The model under review builds one solid part; all positions refer to its coordinate system, in mm. A direction names the side the tool comes from. Coordinates: 2 decimals unless noted, no trailing zeros. Loops run counter-clockwise (first coordinate to the right, second up) from the corner with the lowest first, then second, coordinate; pieces in that order, holes last. Notation, with made-up numbers: (-11, 19.5) - (25, 19.5) arc R22 ccw to (25, 29.5) - close; hole circle Ø6 at (20.5, -18). An arc over 180 degrees is marked (long way). Use a Markdown table: item, result. Add a question column.
1) To check wall thickness, follow L1, parallel to Y at x = 0, z = 41.5; L2, parallel to Z at x = -29, y = 24; L3, parallel to X at y = -3.5, z = 76. State the ranges of each line that lie inside material, in increasing order. Write a range as [from, to].
2) Add section C-C, the plane y = -35. Give the boundary of the cut face in (x, z), and give its area (3 significant figures).
3) For faces 1 (the cylindrical face through (-32.798, 30.075, 62.84)), 2 (the flat face through (9, -19, 0)), list the 3-axis set-ups (+Z, -Z, +X, -X, +Y, -Y) from which the entire face can be reached by the end or side of a thin tool; tool diameter is ignored.
4) Add section D-D, the plane z = 34.5. Give the boundary of the cut face in (x, y), and give its area (3 significant figures).
5) Clearance check with flat-ended pins moving along their axes: pin 1 (1.5 mm diameter, centred on x = -23.5, y = 25, fed in from +Z); pin 2 (6 mm diameter, centred on x = 14, z = 45.5, fed in from -Y); pin 3 (12 mm diameter, centred on x = 35.5, z = 55, fed in from +Y). State where each tip first meets the part, or that it passes through.
6) Add section A-A, the plane x = 0. Give the boundary of the cut face in (y, z), and give its area (3 significant figures).
```python
from build123d import *

# Parameters (mm, degrees)
F0_R        = 45
F0_R_2      = 20
F1_DEPTH    = 2
F1_FACE_R   = 45
F1_FACE_R_2 = 20
F2_DEPTH    = 120
F3_R        = 44.5
F4_DEPTH    = 120


with BuildPart() as f1:
    # F0 (on Top) → F1 (new body)
    with BuildSketch(Plane.XY):
        Circle(F0_R)
        Circle(F0_R_2, mode=Mode.SUBTRACT)
    extrude(amount=F1_DEPTH)

    # F1_face (on face) → F2 (join)
    with BuildSketch(Plane.XY.offset(2)):
        Circle(F1_FACE_R)
        Circle(F1_FACE_R_2, mode=Mode.SUBTRACT)
    extrude(amount=F2_DEPTH)

    # F3 (on face) → F4 (cut)
    with BuildSketch(Plane.XY.offset(122)):
        Circle(F3_R)
    extrude(amount=-F4_DEPTH, mode=Mode.SUBTRACT)


solid = f1.part
```
From the geometry:
| question | item | result |
|---|---|---|
| 1 | L1 | y = [-45, -44.5], [44.5, 45] |
| 1 | L2 | z = [0, 2] |
| 1 | L3 | x = [-44.86, -44.36], [44.36, 44.86] |
| 2 | outline | (-28.28, 0) - (28.28, 0) - (28.28, 122) - (27.48, 122) - (27.48, 2) - (-27.48, 2) - (-27.48, 122) - (-28.28, 122) - close |
| 2 | area | 306 mm^2 |
| 3 | face 1 | +Z |
| 3 | face 2 | -Z, +X, -X, +Y, -Y |
| 4 | outline | circle Ø90 at (0, 0); hole circle Ø89 at (0, 0) |
| 4 | area | 141 mm^2 |
| 5 | pin 1 | stops at z = 2 |
| 5 | pin 2 | stops at y = -43.63 |
| 5 | pin 3 | stops at y = 33.98 |
| 6 | outline | (-45, 0) - (-20, 0) - (-20, 2) - (-44.5, 2) - (-44.5, 122) - (-45, 122) - close; (20, 0) - (45, 0) - (45, 122) - (44.5, 122) - (44.5, 2) - (20, 2) - close |
| 6 | area | 220 mm^2 |
